from build123d import *

# Parameters (mm, degrees)
F0_R      = 25
F1_DEPTH  = 25
F2_R      = 22.5
F3_DEPTH  = 30
F5_W      = 17
F5_H      = 5
F6_DEPTH  = 10
F7_R      = 0.9
F8_DEPTH  = 1
F9_W      = 0.4566367716
F9_H      = 0.1114215702
F9_W_2    = 0.1583136618
F9_H_2    = 0.5275197327
F9_W_3    = 0.4842821509
F9_H_3    = 0.4520714283
F10_DEPTH = 0.2
F11_W     = 0.1633954234
F11_H     = 0.5346611142
F11_W_2   = 0.5340673961
F11_H_2   = 0.1833848655
F11_W_3   = 0.5863611586
F11_H_3   = 0.598071143
F12_DEPTH = 0.2
F13_R     = 0.9
F14_DEPTH = 1
F16_W     = 0.1523271203
F16_H     = 0.6093140692
F16_H_2   = 0.1280289143
F16_W_2   = 0.5286876112
F16_W_3   = 0.605950132
F16_H_3   = 0.6601605564
F17_DEPTH = 0.2
F15_W     = 0.1208484173
F15_H     = 0.469468534
F15_H_2   = 0.0698883086
F15_W_2   = 0.0528423116
F15_H_3   = 0.1033879817
F15_W_3   = 0.0704331324
F15_W_4   = 0.469468534
F15_H_4   = 0.5403161049
F15_W_5   = 0.5258051679
F18_DEPTH = 0.2
F19_W     = 20.6024695653
F19_H     = 7.5707876822
F19_W_2   = 17
F19_H_2   = 5
F20_DEPTH = 25


with BuildPart() as f1:
    # F0 (on Right) → F1 (new body)
    with BuildSketch(Plane.YZ):
        Circle(F0_R)
    extrude(amount=F1_DEPTH)

    # F2 (on face) → F3 (cut)
    with BuildSketch(Plane.YZ.offset(25)):
        Circle(F2_R)
    extrude(amount=-F3_DEPTH, mode=Mode.SUBTRACT)

    # F5 (on offset) → F6 (join)
    with BuildSketch(Plane.XY.offset(23)):
        with Locations((12.5475367568, 3.0585098453)):
            Rectangle(F5_W, F5_H)
    extrude(amount=F6_DEPTH)

    # F7 (on face) → F8 (join)
    with BuildSketch(Plane(origin=(0, 5.5585098453, 0), x_dir=(-1, 0, 0), z_dir=(0, 1, 0))):
        with Locations((-19.3896782356, 25.9250514209)):
            Circle(F7_R)
        with Locations((-5.5436493817, 25.9250514209)):
            Circle(F7_R)
    extrude(amount=F8_DEPTH)

    # F9 (on face) → F10 (cut)
    with BuildSketch(Plane(origin=(0, 6.5585098453, 0), x_dir=(-1, 0, 0), z_dir=(0, 1, 0))):
        with Locations((-19.6518069133, 25.9384280071)):
            Rectangle(F9_W, F9_H)
        with Locations((-19.3443316966, 25.9384280071)):
            Rectangle(F9_W_2, F9_H)
        with Locations((-19.3443316966, 25.6189573556)):
            Rectangle(F9_W_2, F9_H_2)
        with Locations((-19.0230337903, 25.9384280071)):
            Rectangle(F9_W_3, F9_H)
        with Locations((-19.3443316966, 26.2201745063)):
            Rectangle(F9_W_2, F9_H_3)
    extrude(amount=-F10_DEPTH, mode=Mode.SUBTRACT)

    # F11 (on face) → F12 (cut)
    with BuildSketch(Plane(origin=(0, 6.5585098453, 0), x_dir=(-1, 0, 0), z_dir=(0, 1, 0))):
        with Locations((-5.5837228429, 25.5438815802)):
            Rectangle(F11_W, F11_H)
        with Locations((-5.9324542526, 25.9029045701)):
            Rectangle(F11_W_2, F11_H_2)
        with Locations((-5.5837228429, 25.9029045701)):
            Rectangle(F11_W, F11_H_2)
        with Locations((-5.2088445518, 25.9029045701)):
            Rectangle(F11_W_3, F11_H_2)
        with Locations((-5.5837228429, 26.2936325744)):
            Rectangle(F11_W, F11_H_3)
    extrude(amount=-F12_DEPTH, mode=Mode.SUBTRACT)

    # F13 (on face) → F14 (join)
    with BuildSketch(Plane.XZ.offset(-0.5585098453)):
        with Locations((6.0973112057, 26.2796394527)):
            Circle(F13_R)
        with Locations((18.8313634067, 26.2796394527)):
            Circle(F13_R)
    extrude(amount=F14_DEPTH)

    # F16 (on face) → F17 (cut)
    with BuildSketch(Plane.XZ.offset(0.4414901547)):
        with Locations((18.7808908522, 26.6468180344)):
            Rectangle(F16_W, F16_H)
        with Locations((18.7808908522, 26.2781465426)):
            Rectangle(F16_W, F16_H_2)
        with Locations((18.4403834864, 26.2781465426)):
            Rectangle(F16_W_2, F16_H_2)
        with Locations((19.1600294784, 26.2781465426)):
            Rectangle(F16_W_3, F16_H_2)
        with Locations((18.7808908522, 25.8840518072)):
            Rectangle(F16_W, F16_H_3)
    extrude(amount=-F17_DEPTH, mode=Mode.SUBTRACT)

    # F15 (on face) → F18 (cut)
    with BuildSketch(Plane.XZ.offset(0.4414901547)):
        with Locations((6.0697374865, 26.6739912331)):
            Rectangle(F15_W, F15_H)
        with Locations((6.0697374865, 26.4043128118)):
            Rectangle(F15_W, F15_H_2)
        with Locations((5.9828921221, 26.3176746666)):
            Rectangle(F15_W_2, F15_H_3)
        with Locations((6.0697374865, 26.3176746666)):
            Rectangle(F15_W, F15_H_3)
        with Locations((6.1653782614, 26.3176746666)):
            Rectangle(F15_W_3, F15_H_3)
        with Locations((5.7217366993, 26.3176746666)):
            Rectangle(F15_W_4, F15_H_3)
        with Locations((6.0697374865, 25.9958226234)):
            Rectangle(F15_W, F15_H_4)
        with Locations((6.4634974115, 26.3176746666)):
            Rectangle(F15_W_5, F15_H_3)
    extrude(amount=-F18_DEPTH, mode=Mode.SUBTRACT)

    # F19 (on face) → F20 (join)
    with BuildSketch(Plane.XY.offset(33)):
        with Locations((12.5949246576, 2.9163391446)):
            Rectangle(F19_W, F19_H)
        with Locations((12.5475367568, 3.0585098453)):
            Rectangle(F19_W_2, F19_H_2, mode=Mode.SUBTRACT)
        with Locations((12.5475367568, 3.0585098453)):
            Rectangle(F19_W_2, F19_H_2)
    extrude(amount=F20_DEPTH)


solid = f1.part
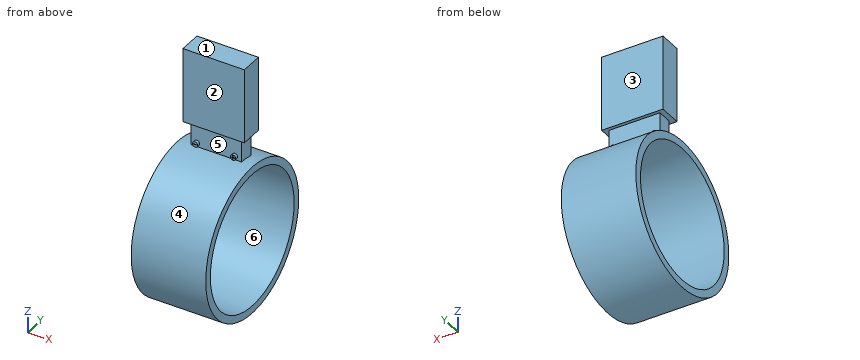
The model under review builds one solid part; all positions refer to its coordinate system, in mm. Face numbers are marked on the shaded views. A direction names the side the tool comes from. Round coordinates to 2 decimals unless told otherwise and drop trailing zeros. Write each loop counter-clockwise with the first axis right and the second up, starting at its lowest first coordinate (ties: lowest second). Pieces come first, ordered by that corner, then holes. Notation, with made-up numbers: M 81.5,25 L 92.5,25 A11 cw 92.5,40 Z; hole C 69.5,82.5 d10. An arc over 180 degrees is marked long. Use a Markdown table: item, result. Add a question column.
Q1. We need section C-C, the plane y = -6.5. State the section outline as (x, z) points.
Q2. We need section B-B, the plane x = 8.75. State the section outline as (y, z) points, plus the area to 3 significant figures.
Q3. The part is to be moulded in two halves that separate along Y. For the marked faces 4, 5 and 6, say which applies: pulls with the +Y half, pulls with the -Y half, needs draft (parallel to the pull), parting line crosses it, or undercut.
Q4. We need section D-D, the plane z = 29.5. State the section outline as (x, y) points, plus the area to 3 significant figures.
Q5. Insertion check: pin 1 (1 mm diameter, centred on x = 6, z = 25.5, fed in from +Y); pin 2 (0.9 mm diameter, centred on x = 6, z = 26, fed in from -Y); pin 3 (10 mm diameter, centred on y = 8, z = 35.5, fed in from +X). Each pin has a flat end and moves straight along its axis. Give the tip position at first contact, or say it passes through.
Q6. We need section A-A, the plane z = 0. State the section outline as (x, y) points, plus the area to 3 significant figures.
Q7. Machinability: for the marked faces 1, 2 and 3, which of the approach directions +Z, -Z, +X, -X, +Y, -Y give a long, thin tool a straight path to every point of the face, cutting with its end or side? Answer none if there is none.
Q8. To check wall thickness, follow line 1 (Z direction, x = 14.25, y = 0); line 2 (Z direction, x = 19.5, y = 0); line 3 (Y direction, x = 8, z = 49.5). State the ranges of each line that lie inside material, in increasing order.
Findings below:
| question | item | result |
|---|---|---|
| 1 | outline | M 0,-24.14 L 25,-24.14 L 25,-21.54 L 0,-21.54 Z; M 0,21.54 L 25,21.54 L 25,24.14 L 0,24.14 Z |
| 2 | outline | M -0.87,33 L 0.56,33 L 0.56,24.99 A25 ccw long 5.56,24.37 L 5.56,33 L 6.7,33 L 6.7,58 L -0.87,58 Z; hole C 0,0 d45 |
| 2 | area | 603 mm² |
| 3 | face 4 | parting line crosses it |
| 3 | face 5 | pulls with the -Y half |
| 3 | face 6 | undercut |
| 4 | outline | M 4.05,0.56 L 21.05,0.56 L 21.05,5.56 L 4.05,5.56 Z |
| 4 | area | 85.0 mm² |
| 5 | pin 1 | stops at y = 6.56 |
| 5 | pin 2 | stops at y = -0.44 |
| 5 | pin 3 | stops at x = 22.9 |
| 6 | outline | M 0,-25 L 25,-25 L 25,-22.5 L 0,-22.5 Z; M 0,22.5 L 25,22.5 L 25,25 L 0,25 Z |
| 6 | area | 125 mm² |
| 7 | face 1 | +Z, +X, -X, +Y, -Y |
| 7 | face 2 | +Z, +X, -X, -Y |
| 7 | face 3 | +Z, +X, -X, +Y |
| 8 | line 1 | z = -25 to -22.5, 22.5 to 25, 33 to 58 |
| 8 | line 2 | z = -25 to -22.5, 22.5 to 25, 25.68 to 26.88, 33 to 58 |
| 8 | line 3 | y = -0.87 to 6.7 |
